Input: part model. Units: mm. Frame: model coordinates. Face numbers are marked on the shaded views. A direction names the side the tool comes from. Coordinates: 2 decimals unless noted, no trailing zeros. Order: outer loops, then holes, each group sorted by start corner. A loop starts at its lowest first (then second) coordinate and runs counter-clockwise, first axis right, second up. Notation, with made-up numbers: (37, 37) - (87, 37) arc R31 cw to (87, 76) - close; hole circle Ø6 at (-38, 7). An arc over 180 degrees is marked (long way). One line per question, with ' | ' between items.
Autodesk Fusion 360 part; units mm, degrees
sketch "Sketch1" plane through (0, 0, 0) normal (0, 0, 1) x (1, 0, 0)
  line L0 (0, 0) -> (-34, 0)
  line L1 (-34, 42) -> (0, 42)
  line L2 (0, 42) -> (0, 0)
  line L3 (-34, -3) -> (-34, 45)
  line L4 (3, -3) -> (-34, -3)
  line L5 (-34, 45) -> (3, 45)
  line L6 (3, 45) -> (3, -3)
  line L7 (-18, 55) -> (-16, 55)
  line L8 (-12, 51) -> (-12, 45)
  line L9 (-12, 45) -> (-22, 45)
  line L10 (-22, 45) -> (-22, 51)
  circle A0 centre (-17, 50) radius 1.75
  arc A1 (-18, 55) -> (-22, 51) centre (-18, 51) ccw
  arc A2 (-12, 51) -> (-16, 55) centre (-16, 51) ccw
  circle A3 centre (-17, -8) radius 1.75
  line L11 (-22, -3) -> (-22, -9)
  arc A4 (-22, -9) -> (-18, -13) centre (-18, -9) ccw
  line L12 (-18, -13) -> (-16, -13)
  arc A5 (-16, -13) -> (-12, -9) centre (-16, -9) ccw
  line L13 (-12, -9) -> (-12, -3)
  line L14 (3, 45) -> (-14.0543, 54.4949)
  line L15 (3, -3) -> (-14.0543, -12.4949)
  line L16 (-34, 45) -> (-20.2422, 54.3125)
  line L17 (-34, -3) -> (-20.2422, -12.3125)
  line L18 (-19.75, -9.5877) -> (-17, -11.1754)
  line L19 (-17, -11.1754) -> (-14.25, -9.5877)
  line L20 (-14.25, -9.5877) -> (-14.25, -6.4123)
  line L21 (-14.25, -6.4123) -> (-17, -4.8246)
  line L22 (-17, -4.8246) -> (-19.75, -6.4123)
  line L23 (-19.75, -6.4123) -> (-19.75, -9.5877)
  point P0 (-22, 55)
  point P1 (-12, 55)
  point P2 (-17, -8)
  dimension "d1" = 34
  dimension "d2" = 42
  dimension "d6" = 10
  dimension "d7" = 10
  dimension "d8" = 3.5
  dimension "d9" = 4
  dimension "d24" = 20
  dimension "d43" = 5
  dimension "d79" = 2.75
extrude "Extrude1" add sketch "Sketch1" along normal blind 11 contours L0 L1 L2 L3 L4 L5 L6 L9
extrude "Extrude2" add sketch "Sketch1" along normal blind 3 from surface at 8 contours L4 L11 A4 L17 | L4 L11 A4 L12 A5 L13 | L5 L10 A1 L16 | L4 A5 L13 L15 | L5 L7 L8 L9 L10 A1 A2 | L5 L8 A2 L14 | L18 L19 L20 L21 L22 L23
extrude "Extrude5" add sketch "Sketch1" along normal blind 3 contours L0 L1 L2 L3
ref_plane "WorkPlane3" through (0, 21, 0) normal (0, 1, 0) x (0, 0, 1)
sketch "Sketch5" plane through (0, 0, 3) normal (0, 0, 1) x (-1, 0, 0)
  line L0 (30, 0) -> (30, -42)
  line L1 (34, -42) -> (34, 0)
  line L2 (34, 0) -> (0, 0)
  line L3 (0, 0) -> (0, -42)
  line L4 (0, -42) -> (34, -42)
  line L5 (34, -42) -> (34, 0)
  line L6 (0, -21) -> (17, 0)
  line L7 (0, -42) -> (30, -4.9412)
  line L8 (17, -42) -> (30, -25.9412)
  line L9 (17, -42) -> (0, -21)
  line L10 (0, 0) -> (30, -37.0588)
  line L11 (30, -16.0588) -> (17, 0)
  line L12 (18.1659, -41.0562) -> (1.1659, -20.0562)
  line L13 (15.0701, -42) -> (0, -23.384)
  line L14 (1.9299, -42) -> (30, -7.3252)
  line L15 (0, -39.616) -> (30, -2.5572)
  line L16 (18.9299, -42) -> (30, -28.3252)
  line L17 (15.8341, -41.0562) -> (30, -23.5572)
  line L18 (1.1659, -21.9438) -> (18.1659, -0.9438)
  line L19 (0, -18.616) -> (15.0701, 0)
  line L20 (0, -2.384) -> (30, -39.4428)
  line L21 (1.9299, 0) -> (30, -34.6748)
  line L22 (30, -13.6748) -> (18.9299, 0)
  line L23 (30, -18.4428) -> (15.8341, -0.9438)
  dimension "d64" = 42
  dimension "d65" = 4
  dimension "d66" = 1.5
  dimension "d72" = 1.5
extrude "Extrude6" cut sketch "Sketch5" against normal blind 5 contours L0 L2 L15 L22 | L0 L14 L22 | L0 L4 L16 L20 | L2 L19 L21 | L15 L18 L21 L23 | L0 L14 L17 L21 L23 | L0 L16 L21 | L4 L13 L14 | L3 L19 L20 | L12 L15 L18 L20 | L12 L14 L17 L20 | L3 L13 L15
sketch "Sketch6" plane through (-34, 0, 0) normal (-1, 0, 0) x (0, -1, 0)
  line L0 (-45, 0) -> (3, 0)
  line L1 (3, 0) -> (3, 8)
  line L2 (3, 8) -> (3, 11)
  line L3 (3, 11) -> (0, 11)
  line L4 (0, 11) -> (0, 3)
  line L5 (0, 3) -> (-42, 3)
  line L6 (-42, 3) -> (-42, 11)
  line L7 (-42, 11) -> (-45, 11)
  line L8 (-45, 11) -> (-45, 8)
  line L9 (-45, 8) -> (-45, 0)
  line L10 (3, 8) -> (12.3125, 8)
  line L11 (3, 0) -> (3, 8)
  line L12 (9.5141, 8) -> (3, 2.5254)
extrude "Extrude8" add sketch "Sketch6" against normal blind 3 from surface at -10 contours L1 L10 L11 L12
ref_plane "WorkPlane4" through (-17, 21, 5.5) normal (-1, 0, 0) x (0, -1, 0)
mirror "Mirror4" about plane through (-17, 21, 5.5) normal (-1, 0, 0) of "Extrude8"
mirror "Mirror5" about plane through (0, 21, 0) normal (0, 1, 0) of "Mirror4", "Extrude8"
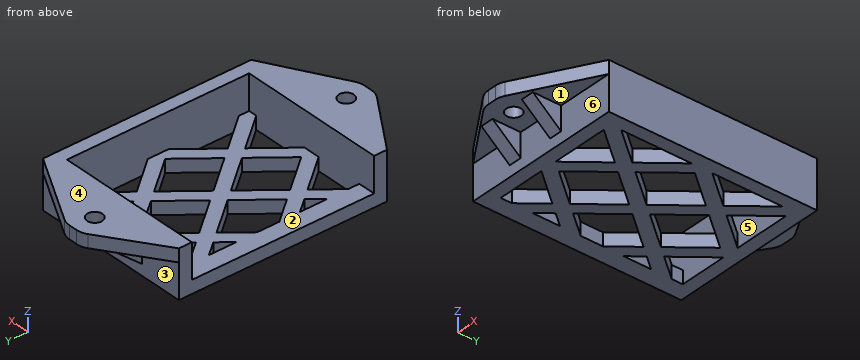
Item 1: Draft query along Y for the marked faces 4, 5 and 6. Return one class per face: released by +Y, released by -Y, zero draft, split by the parting line, or undercut.
Data:
face 4: zero draft | face 5: undercut | face 6: released by -Y
Item 2: Section C-C on x = -22. Count the separate pieces of the cut face and the enclosed holes in it, and give its area (3 significant figures).
Data:
separate pieces: 6 | enclosed holes: 0 | area: 208 mm^2
Item 3: Access query for the marked faces 1, 2 and 3. Directions: +Z, -Z, +X, -X, +Y, -Y. A direction counts if a zero-diameter tool reaches every point of the face in a straight line with its end or side. Return the directions, or none.
Data:
face 1: -Z, -Y | face 2: +Z, -X | face 3: -Z, +Y
Item 4: Section B-B on y = 19.5. Return the cut outline in (x, z).
Data:
outline: (-34, 0) - (-30, 0) - (-30, 3) - (-34, 3) - close; (-20.14, 0) - (-13.86, 0) - (-13.86, 3) - (-20.14, 3) - close; (-3.14, 0) - (3, 0) - (3, 11) - (0, 11) - (0, 3) - (-3.14, 3) - close
Item 5: Section D-D on y = 4.5. Return the cut outline in (x, z).
Data:
outline: (-34, 0) - (-28.43, 0) - (-28.43, 3) - (-34, 3) - close; (-22.57, 0) - (-18.71, 0) - (-18.71, 3) - (-22.57, 3) - close; (-15.29, 0) - (-11.43, 0) - (-11.43, 3) - (-15.29, 3) - close; (-5.57, 0) - (-1.71, 0) - (-1.71, 3) - (-5.57, 3) - close; (0, 0) - (3, 0) - (3, 11) - (0, 11) - close
Item 6: Section A-A on z = 9.5. Return the cut outline in (x, y).
Data:
outline: (-34, -3) - (-20.24, -12.31) arc R4 ccw to (-18, -13) - (-16, -13) arc R4 ccw to (-14.05, -12.49) - (3, -3) - (3, 45) - (-14.05, 54.49) arc R4 ccw to (-16, 55) - (-18, 55) arc R4 ccw to (-20.24, 54.31) - (-34, 45) - (-34, 42) - (0, 42) - (0, 0) - (-34, 0) - close; hole circle Ø3.5 at (-17, -8); hole circle Ø3.5 at (-17, 50)
Item 7: Ray query, line 1 (Y direction, x = -17, z = 9.4); line 2 (Y direction, x = -25, z = 5.5); line 3 (X direction, y = 4, z = 0.5). Return the intervals inside material, ascending.
Data:
line 1: -13 to -9.75, -6.25 to 0, 42 to 48.25, 51.75 to 55 | line 2: -3 to 0, 42 to 45 | line 3: -34 to -28.83, -22.17 to -18.31, -15.69 to -11.83, -5.17 to -1.31, 0 to 3
Item 8: Contact query for flat-ended pins moving along their axis: P1, Ø1, axis at y = 32, z = 9, coming from the -X side; P2, Ø4.5, axis at y = -5.5, z = 4, coming from the -X side; P3, Ø5.5, axis at x = -16, z = 3.5, coming from the -Y side. Output: stop coordinate, or through.
Data:
P1: x = 0 | P2: x = -24 | P3: y = -3
